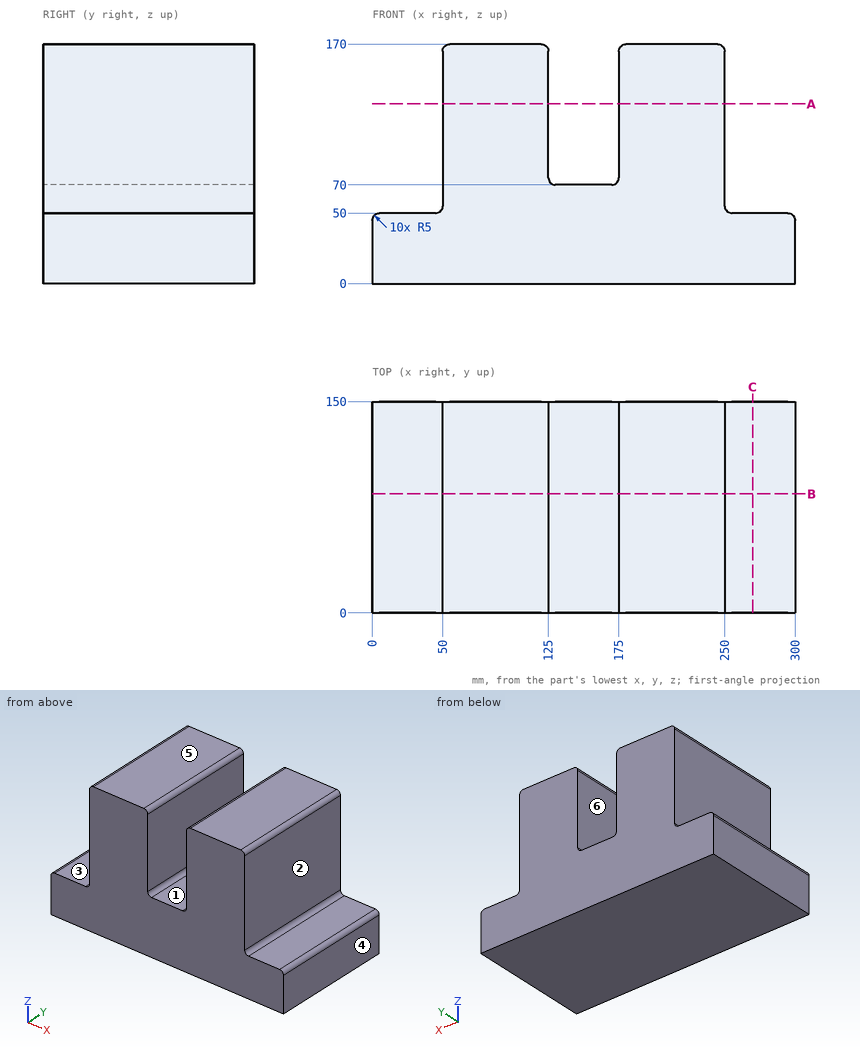
Design review of the part shown in the three views and the two pictorial views. Dimensions are in mm from the part's minimum x, y and z. A direction names the side the tool comes from. Round coordinates to 2 decimals unless told otherwise and drop trailing zeros. Loops run counter-clockwise (first coordinate to the right, second up) from the corner with the lowest first, then second, coordinate; pieces in that order, holes last. Notation, with made-up numbers: M -38,-32 L -3,-32 A9 cw -3,-25 Z; hole C 45.5,-26 d11. An arc over 180 degrees is marked long. Put each result on its own line as item: value.
Q1. Consider section C-C, the plane x = 270. Give the boundary of the cut face in (y, z).
Result set:
outline: M 0,0 L 150,0 L 150,50 L 0,50 Z
Q2. Machinability: for the marked faces 1, 2 and 3, which of the approach directions +Z, -Z, +X, -X, +Y, -Y give a long, thin tool a straight path to every point of the face, cutting with its end or side? Answer none if there is none.
Result set:
face 1: +Z, +Y, -Y
face 2: +Z, +X, +Y, -Y
face 3: +Z, -X, +Y, -Y
Q3. To check wall thickness, follow L1, parallel to X at y = 44, z = 128.5; L2, parallel to Z at x = 263, y = 89; L3, parallel to X at y = 37, z = 59. State the ranges of each line that lie inside material, in increasing order.
Result set:
L1: x = 50 to 125, 175 to 250
L2: z = 0 to 50
L3: x = 50 to 250
Q4. Mouldability with a two-part tool opening along X and no side actions: class the marked faces 4, 5 and 6 as released by +X, released by -X, zero draft, split by the parting line, or undercut.
Result set:
face 4: released by +X
face 5: zero draft
face 6: undercut
Q5. For pin 1 (6 mm diameter, centred on y = 17.5, z = 59, fed in from -X), flat-tipped, find the tip position at first contact; note if it passes through.
Result set:
pin 1: stops at x = 50
Q6. Consider section B-B, the plane y = 84.5. Give the boundary of the cut face in (x, z), then the cut area to 3 significant figures.
Result set:
outline: M 0,0 L 300,0 L 300,45 A5 ccw 295,50 L 255,50 A5 cw 250,55 L 250,165 A5 ccw 245,170 L 180,170 A5 ccw 175,165 L 175,75 A5 cw 170,70 L 130,70 A5 cw 125,75 L 125,165 A5 ccw 120,170 L 55,170 A5 ccw 50,165 L 50,55 A5 cw 45,50 L 5,50 A5 ccw 0,45 Z
area: 34,000 mm²
Q7. Consider section A-A, the plane z = 127.5. Give the boundary of the cut face in (x, y).
Result set:
outline: M 50,0 L 125,0 L 125,150 L 50,150 Z; M 175,0 L 250,0 L 250,150 L 175,150 Z
